Check sheet for the drawn part. Datum: minimum x, y, z corner. Units: mm. A direction names the side the tool comes from. Give positions to 0.01 mm unless a question says otherwise; leave off trailing zeros. Loops run counter-clockwise (first coordinate to the right, second up) from the corner with the lowest first, then second, coordinate; pieces in that order, holes last. Notation, with made-up numbers: M 65.5,48 L 100.5,48 A7 ccw 100.5,61 Z; hole C 14.5,0.25 d9. An arc over 180 degrees is marked long. Write each question's results on one line, items separated by ' | '. Start each with the question number.
1. Go/stop test with flat-tipped pins: pin 1 (1.6 mm diameter, centred on x = 2, z = 12, fed in from -Y); pin 2 (2.5 mm diameter, centred on x = 3.5, y = 1.5, fed in from -Z). Record where each tip stops, or that it passes through.
2. Sectioned sample at B-B on z = 15.5. Record the cut outline in (x, y) (1 decimal), and give its area (3 significant figures).
3. Sectioned sample at C-C on z = 19. Record the cut outline in (x, y) (1 decimal).
4. Sectioned sample at A-A on y = 61.5. Record the cut outline in (x, z).
5. Material ranges on line 1 along Z through (x, y) = (1, 13); line 2 along Z through (x, y) = (3.25, 9); line 3 along Y through (x, z) = (4.75, 21.25) (3 decimals), recorded low to high.
6. Draft check along Z on the marked faces 1, 2, 3 and 4. Enter one of: pulls with the +Z half, pulls with the -Z half, needs draft (parallel to the pull), parting line crosses it, or undercut.
7. Tool access check on the marked faces 5, 6 and 7. Record the directions out of +Z, -Z, +X, -X, +Y, -Y that give a thin tool (end or side, any length) a straight path to the whole face; none if there is none.
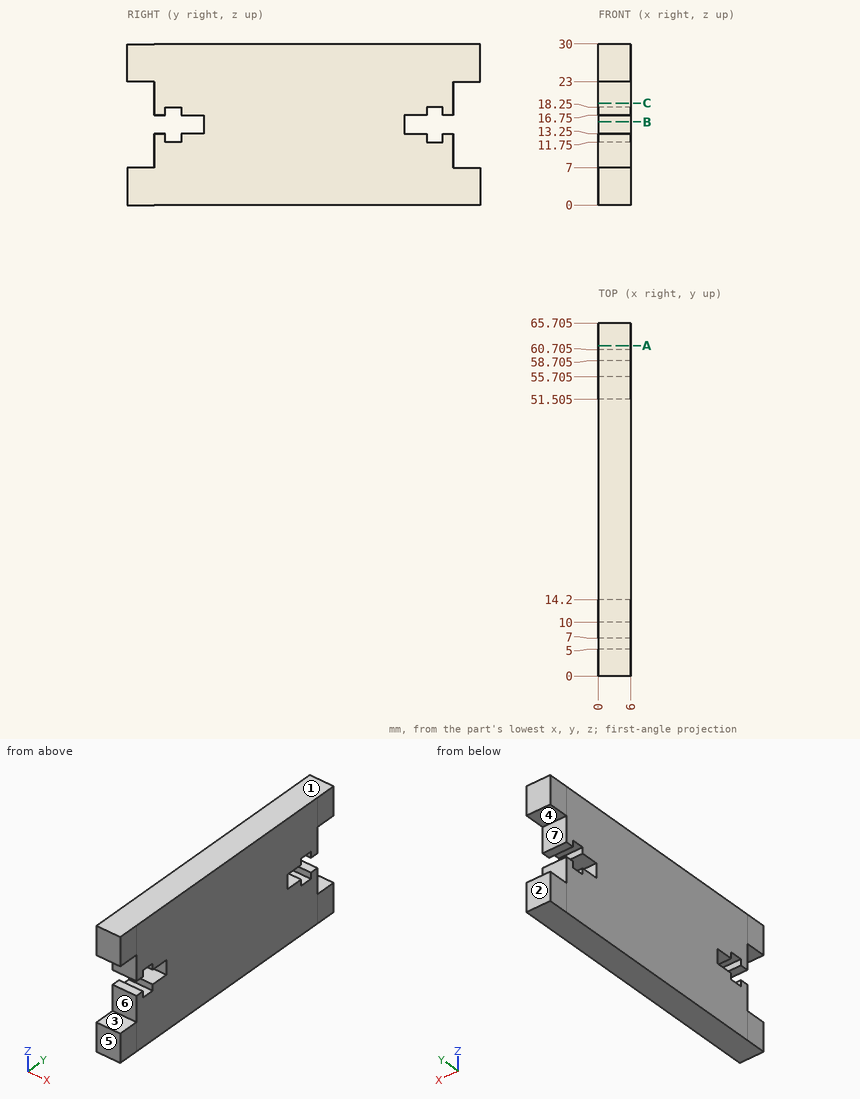
Output values:
1) pin 1: y = 5 | pin 2: z = 0
2) outline: M 0,14.2 L 6,14.2 L 6,51.5 L 0,51.5 Z | area: 224 mm2
3) outline: M 0,5 L 6,5 L 6,60.7 L 0,60.7 Z
4) outline: M 0,0 L 6,0 L 6,7 L 0,7 Z; M 0,23 L 6,23 L 6,30 L 0,30 Z
5) line 1: 0 to 13.25, 16.75 to 30 | line 2: 0 to 11.75, 18.25 to 30 | line 3: 5 to 60.705
6) face 1: pulls with the +Z half | face 2: needs draft | face 3: undercut | face 4: undercut
7) face 5: +Z, -Z, +X, -X, -Y | face 6: +X, -X, -Y | face 7: +X, -X, +Y
